Geometry: final body of the model. Coordinates: model frame, mm. A direction names the side the tool comes from. Give positions to 0.01 mm unless a question says otherwise; leave off trailing zeros. Write each loop counter-clockwise with the first axis right and the second up, starting at its lowest first coordinate (ties: lowest second). Pieces come first, ordered by that corner, then holes. Notation, with made-up numbers: (-5, -10) -> (5, -10) arc R33 ccw to (5, 25) -> close; hole circle Ø8 at (86, -28.5). An arc over 180 degrees is marked (long way). Use CSV: the item, a comma, the result in double quotes. Start each with the question number.
1) Set-up query: faces 5 (the face through (2.8, 0, 9.3)), 6 (the face through (-6.324, 4.535, -4.032)). Return all of +Z, -Z, +X, -X, +Y, -Y with unobstructed straight access to the full face (end or side cutting, diameter ignored); none if empty.
2) Section A-A (z = 0). Output: boundary loops of the cut face in (x, y), plus the area to 3 significant figures.
3) Section B-B (x = 0). Output: boundary loops of the cut face in (y, z).
4) Contact query for flat-ended pins moving along their axis: P1, Ø8, axis at x = -8.5, y = 12, coming from the +Z side; P2, Ø12, axis at x = 1, z = -3, coming from the -Y side; P3, Ø2.5, axis at x = 0.5, z = -1, coming from the -Y side. Output: stop coordinate, or through.
5) Section D-D (y = 11.5). Output: boundary loops of the cut face in (x, z).
6) Material intervals for line 1 (Y direction, x = 5, z = 3.5); line 2 (X direction, y = 5.25, z = -4.5); line 3 (X direction, y = 2.5, z = 6), sorted ascending. Write a range as [from, to].
7) Section C-C (y = 5.75). Output: boundary loops of the cut face in (x, z).
8) Draft query along X for faces 1 (the face through (0, 16, 0)), 2 (the face through (15.793, 7.231, 3.507)), 3 (the face through (-2, 7, 2)), 4 (the face through (-0.1, 9.5, 2.5)). Return one class per face: pulls with the +X half, pulls with the -X half, needs draft (parallel to the pull), parting line crosses it, or undercut.
```python
from build123d import *

# Parameters (mm, degrees)
REDONDEO1_R = 2


with BuildPart() as part:
    # Croquis1 → Revolución1 (revolve)
    with BuildSketch(Plane(origin=(0, 0, 0), x_dir=(0, 0, -1), z_dir=(1, 0, 0)), mode=Mode.PRIVATE) as revoluci_n1_sk:
        Polygon((0, 16), (-17, 16), (-15.5, 0), (-7.5, 0), (-7.5, 7), (-2.5, 7), (-2.5, 12), (0, 12), align=None)
    revolve(revoluci_n1_sk.sketch.rotate(Axis((0, 0, 0), (0, 1, 0)), 180), axis=Axis((0, 0, 0), (0, 1, 0)))

    # Redondeo1
    redondeo1_edges = [part.edges().sort_by_distance(p)[0] for p in [
        (0, 0, 7.5),
        (0, 0, 15.5),
    ]]
    fillet(redondeo1_edges, radius=REDONDEO1_R)


solid = part.part
```
Answers follow:
1,face 5,"+Z, -Z, +X, -X, -Y"
1,face 6,"-Y"
2,outline,"(-17, 16) -> (-15.67, 1.81) arc R2 ccw to (-13.68, 0) -> (-9.5, 0) arc R2 ccw to (-7.5, 2) -> (-7.5, 7) -> (-2.5, 7) -> (-2.5, 12) -> (2.5, 12) -> (2.5, 7) -> (7.5, 7) -> (7.5, 2) arc R2 ccw to (9.5, 0) -> (13.68, 0) arc R2 ccw to (15.67, 1.81) -> (17, 16) -> close"
2,area,"387 mm^2"
3,outline,"(0, -13.68) arc R2 ccw to (1.81, -15.67) -> (16, -17) -> (16, 17) -> (1.81, 15.67) arc R2 ccw to (0, 13.68) -> (0, 9.5) arc R2 ccw to (2, 7.5) -> (7, 7.5) -> (7, 2.5) -> (12, 2.5) -> (12, -2.5) -> (7, -2.5) -> (7, -7.5) -> (2, -7.5) arc R2 ccw to (0, -9.5) -> close"
4,P1,"stops at z = 16.07"
4,P2,"stops at y = 0.03"
4,P3,"stops at y = 12"
5,outline,"circle Ø33.16 at (0, 0); hole circle Ø5 at (0, 0)"
6,line 1,"y = [7, 16]"
6,line 2,"x = [-15.35, -6], [6, 15.35]"
6,line 3,"x = [-14.55, -4.5], [4.5, 14.55]"
7,outline,"circle Ø32.08 at (0, 0); hole circle Ø15 at (0, 0)"
8,face 1,"needs draft"
8,face 2,"parting line crosses it"
8,face 3,"undercut"
8,face 4,"undercut"
